Could you check a few things on this model? Use its own coordinates, in mm. Give positions to 0.01 mm unless a question says otherwise; leave off trailing zeros. Order: outer loops, then holes, each group sorted by start corner. A loop starts at its lowest first (then second) coordinate and runs counter-clockwise, first axis right, second up.
(1) Will these pins go through, and if not, where does the flat tip stop? pin 1 (3 mm diameter, centred on y = 151, z = 40, fed in from -X); pin 2 (8 mm diameter, centred on x = -390, z = 33.5, fed in from -Y); pin 3 (15 mm diameter, centred on y = 580, z = 26, fed in from +X).
(2) Imagine slicing it at C-C, the plane x = -180.5. Write out the boundary of the cut face in (y, z).
(3) Imagine slicing it at B-B, the plane y = 104. Write out the boundary of the cut face in (x, z).
(4) If I drill on probe 1 along X at (y, z) = (264, 22.5); probe 2 along Y at (x, z) = (-36, 37); probe 3 along Y at (x, z) = (-49, 45.5), over which ranges is the centre line in solid material (lowest first)?
(5) Imagine slicing it at A-A, the plane x = -68. Write out the boundary of the cut face in (y, z), then the cut area to 3 significant figures.
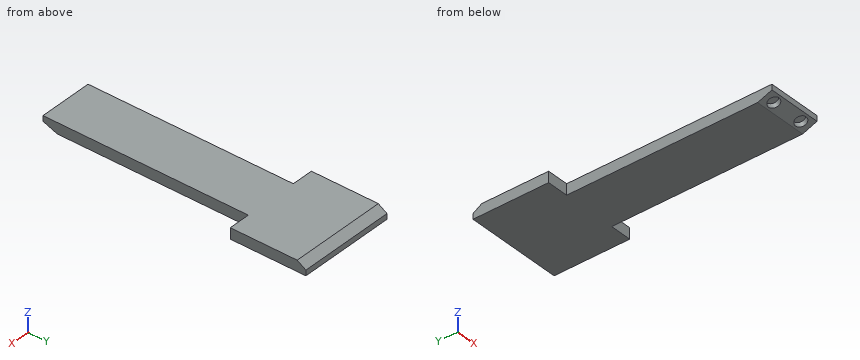
from build123d import *

# Parameters (mm, degrees)
F0_W     = 450
F0_H     = 1300
F1_DEPTH = 50
F2_W     = 100
F2_H     = 950
F3_DEPTH = 50.001
F5_DEPTH = 350.001
F7_DEPTH = 450.001
F8_R     = 26
F9_DEPTH = 25


with BuildPart() as f1:
    # F0 (on Top) → F1 (new body)
    with BuildSketch(Plane.XY):
        with Locations((-215.0315403938, 604.3549530208)):
            Rectangle(F0_W, F0_H)
    extrude(amount=F1_DEPTH)

    # F2 (on face) → F3 (cut, through all)
    with BuildSketch(Plane.XY.offset(50)):
        with Locations((-390.0315403938, 429.3549530208)):
            Rectangle(F2_W, F2_H)
        with Locations((-40.0315403938, 429.3549530208)):
            Rectangle(F2_W, F2_H)
    extrude(amount=-F3_DEPTH, mode=Mode.SUBTRACT)

    # F4 (on face) → F5 (cut, through all)
    with BuildSketch(Plane.YZ.offset(-90.0315403938)):
        Polygon((20.675143227, 0), (-45.6450469792, 25), (-45.6450469792, 0), align=None)
    extrude(amount=-F5_DEPTH, mode=Mode.SUBTRACT)

    # F6 (on face) → F7 (cut, through all)
    with BuildSketch(Plane.YZ.offset(9.9684596062)):
        Polygon((1214.1013145447, 50), (1254.3549530208, 25), (1254.3549530208, 50), align=None)
    extrude(amount=-F7_DEPTH, mode=Mode.SUBTRACT)

    # F8 (on face) → F9 (cut)
    with BuildSketch(Plane(origin=(0, 2.5723708618, 6.8240049934), x_dir=(1, 0, 0), z_dir=(0, -0.3527301048, -0.9357251056))):
        with Locations((-140.0315403938, 16.0916092218)):
            Circle(F8_R)
        with Locations((-290.0315403938, 16.0916092218)):
            Circle(F8_R)
    extrude(amount=-F9_DEPTH, mode=Mode.SUBTRACT)


solid = f1.part
Answer block:
1. pin 1: stops at x = -340.03
1. pin 2: stops at y = 904.35
1. pin 3: stops at x = -90.03
2. outline: (-45.65, 25) - (20.68, 0) - (1254.35, 0) - (1254.35, 25) - (1214.1, 50) - (-45.65, 50) - close
3. outline: (-340.03, 0) - (-90.03, 0) - (-90.03, 50) - (-340.03, 50) - close
4. probe 1: x = -340.03 to -90.03
4. probe 2: y = 904.35 to 1235.03
4. probe 3: y = 904.35 to 1221.35
5. outline: (904.35, 0) - (1254.35, 0) - (1254.35, 25) - (1214.1, 50) - (904.35, 50) - close
5. area: 17,000 mm2
